```python
from build123d import *

# Parameters (mm, degrees)
F0_W     = 2.3575491577
F0_H     = 19.056274371
F0_W_2   = 4.1343827633
F1_DEPTH = 0.8


with BuildPart() as f1:
    # F0 (on Front) → F1 (new body)
    with BuildSketch(Plane.XZ):
        with BuildLine():
            ThreePointArc((0.5134190636, 20.3306143382), (0, 20.3072495762), (-0.5134190636, 20.3306143382))
            Line((-0.5134190636, 20.3306143382), (-11.4882850616, 20.3306143382))
            Line((-11.4882850616, 20.3306143382), (-11.4882850616, -93.387475984))
            Line((-11.4882850616, -93.387475984), (-4.4247405394, -93.387475984))
            Line((-4.4247405394, -93.387475984), (-4.4247405394, -74.3312016129))
            Line((-4.4247405394, -74.3312016129), (-4.4247405394, 7.7945953777))
            Line((-4.4247405394, 7.7945953777), (-2.0671913816, 0))
            Line((-2.0671913816, 0), (-2.0671913816, -68.6852410436))
            Line((-2.0671913816, -68.6852410436), (2.0671913816, -68.6852410436))
            Line((2.0671913816, -68.6852410436), (2.0671913816, 0))
            Line((2.0671913816, 0), (4.4247405394, 7.7945953777))
            Line((4.4247405394, 7.7945953777), (4.4247405394, -74.3312016129))
            Line((4.4247405394, -74.3312016129), (4.4247405394, -93.387475984))
            Line((4.4247405394, -93.387475984), (11.4850704372, -93.387475984))
            Line((11.4850704372, -93.387475984), (11.4850704372, 20.3306143382))
            Line((11.4850704372, 20.3306143382), (0.5134190636, 20.3306143382))
        make_face()
        with BuildLine():
            ThreePointArc((0.5134190636, 20.3306143382), (4.1745945423, 22.1487100844), (5.6526372145, 25.9598867907))
            ThreePointArc((5.6526372145, 25.9598867907), (-3.8111767063, 30.134481333), (-0.5134190636, 20.3306143382))
            Line((-0.5134190636, 20.3306143382), (0.5134190636, 20.3306143382))
        make_face()
        with BuildLine():
            Line((0.5134190636, 20.3306143382), (-0.5134190636, 20.3306143382))
            ThreePointArc((-0.5134190636, 20.3306143382), (0, 20.3072495762), (0.5134190636, 20.3306143382))
        make_face()
        with Locations((3.2459659605, -83.8593387985)):
            Rectangle(F0_W, F0_H)
        with Locations((0, -83.8593387985)):
            Rectangle(F0_W_2, F0_H)
        with Locations((-3.2459659605, -83.8593387985)):
            Rectangle(F0_W, F0_H)
    extrude(amount=F1_DEPTH)


solid = f1.part
```
Input: part model. Units: mm. Frame: model coordinates. Coordinates: 2 decimals unless noted, no trailing zeros. Write each loop counter-clockwise with the first axis right and the second up, starting at its lowest first coordinate (ties: lowest second). Pieces come first, ordered by that corner, then holes. Notation, with made-up numbers: (43.25, -19.5) -> (95.25, -19.5) arc R32 ccw to (95.25, 10.5) -> close; hole circle Ø11 at (-25.75, -24.5). An arc over 180 degrees is marked (long way). Answer as a JSON object with one key per item and string values.
1. Material intervals for line 1 (X direction, y = -0.7, z = -63.5); line 2 (Z direction, x = -7.25, y = -0.35); line 3 (Z direction, x = -1.5, y = -0.75), sorted ascending. Write a range as from..to.
Result set:
{"line 1": "x = -11.49..-4.42, -2.07..2.07, 4.42..11.49", "line 2": "z = -93.39..20.33", "line 3": "z = -93.39..-74.33, -68.69..20.33, 20.51..31.41"}
2. Section C-C on y = -0.2. Return the cut outline in (x, z).
Result set:
{"outline": "(-11.49, -93.39) -> (11.49, -93.39) -> (11.49, 20.33) -> (0.51, 20.33) arc R5.65 ccw (long way) to (-0.51, 20.33) -> (-11.49, 20.33) -> close; hole (-4.42, -74.33) -> (4.42, -74.33) -> (4.42, 7.79) -> (2.07, 0) -> (2.07, -68.69) -> (-2.07, -68.69) -> (-2.07, 0) -> (-4.42, 7.79) -> close"}
3. Section D-D on x = -9.25. Return the cut outline in (y, z).
Result set:
{"outline": "(-0.8, -93.39) -> (0, -93.39) -> (0, 20.33) -> (-0.8, 20.33) -> close"}
4. Mould query, pull axis Z, two halves, no side actions, for faces 1 (the face through (-3.26, -0.39, 3.95)), 2 (the face through (0, -0.8, -30)). Classes: released by +Z, released by -Z, zero draft, split by the parting line, or undercut.
Result set:
{"face 1": "undercut", "face 2": "zero draft"}
5. Section A-A on z = -70.5. Return the cut outline in (x, y).
Result set:
{"outline": "(-11.49, -0.8) -> (-4.42, -0.8) -> (-4.42, 0) -> (-11.49, 0) -> close; (4.42, -0.8) -> (11.49, -0.8) -> (11.49, 0) -> (4.42, 0) -> close"}
6. Section B-B on z = -57. Return the cut outline in (x, y).
Result set:
{"outline": "(-11.49, -0.8) -> (-4.42, -0.8) -> (-4.42, 0) -> (-11.49, 0) -> close; (-2.07, -0.8) -> (2.07, -0.8) -> (2.07, 0) -> (-2.07, 0) -> close; (4.42, -0.8) -> (11.49, -0.8) -> (11.49, 0) -> (4.42, 0) -> close"}
